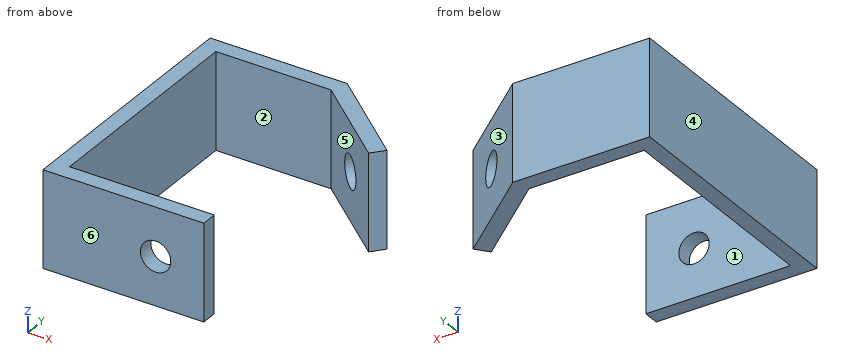
```python
from build123d import *

# Parameters (mm, degrees)
BOSS_EXTRUDE1_DEPTH = 38.1
SKETCH3_R           = 6
CUT_EXTRUDE1_DEPTH  = 23.1
SKETCH4_R           = 6.358205361
CUT_EXTRUDE2_DEPTH  = 23.1


with BuildPart() as part:
    # Sketch2 → Boss-Extrude1 (new body)
    with BuildSketch(Plane.XY):
        Polygon((0, -39.756624631), (63.51, -39.756624631), (63.51, -33.406624631), (6.35, -33.406624631), (6.35, 55.493375369), (51.808789012, 55.493375369), (84.579242619, 27.995699834), (88.66094394, 32.860082048), (54.12, 61.843375369), (0, 61.843375369), align=None)
    extrude(amount=BOSS_EXTRUDE1_DEPTH)

    # Sketch3 → Cut-Extrude1 (cut)
    with BuildSketch(Plane.XZ.offset(39.756624631)):
        with Locations(Location((44.47, 19.05, 0), (0, 0, 270))):
            Circle(SKETCH3_R)
    extrude(amount=-CUT_EXTRUDE1_DEPTH, mode=Mode.SUBTRACT)

    # Sketch4 → Cut-Extrude2 (cut)
    with BuildSketch(Plane(origin=(52.81299808, 62.940080198, 0), x_dir=(0.7660444431189768, -0.6427876096865409, 0), z_dir=(0.6427876096865408, 0.7660444431189767, 0))):
        with Locations(Location((25.986169834, -19.05, 0), (0, 0, 180))):
            Circle(SKETCH4_R)
    extrude(amount=-CUT_EXTRUDE2_DEPTH, mode=Mode.SUBTRACT)


solid = part.part
```
Check sheet for the modelled part. Datum: model origin and axes. Units: mm. Face numbers are marked on the shaded views. A direction names the side the tool comes from. Coordinates: 2 decimals unless noted, no trailing zeros. Loops run counter-clockwise (first coordinate to the right, second up) from the corner with the lowest first, then second, coordinate; pieces in that order, holes last.
1) Release check for a two-part mould opening along Y. For the marked faces 4, 5 and 6 record: released by +Y, released by -Y, zero draft, split by the parting line, or undercut.
2) Access from +Z, -Z, +X, -X, +Y, -Y to the whole of each face (thin tool, end or side, straight path). Record for the marked faces 1, 2 and 3.
3) Material ranges on probe 1 along Y at (x, z) = (51, 13.5); probe 2 along X at (y, z) = (-35, 19.05); probe 3 along Z at (x, y) = (44, -34), recorded low to high.
4) Sectioned sample at B-B (z = 21.5). Record the boundary of the cut face in (x, y) (3 decimals), and give its area (3 significant figures).
5) Sectioned sample at D-D (z = 10). Record the boundary of the cut face in (x, y).
6) Sectioned sample at C-C (y = 35.5). Record the boundary of the cut face in (x, z).
7) Gauge pin test, flat ends, axial feed: pin 1 (8 mm diameter, centred on y = 45, z = 17, fed in from +X); pin 2 (5 mm diameter, centred on y = 47.5, z = 33.5, fed in from -X); pin 3 (1.9 mm diameter, centred on y = -37.5, z = 20, fed in from +X). Record the tip position at first contact, or that the pin passes through.
8) Sectioned sample at A-A (x = 44.47). Record the boundary of the cut face in (y, z), and give its area (3 significant figures).
Check sheet entries:
1. face 4: zero draft
1. face 5: undercut
1. face 6: released by -Y
2. face 1: +Z, -Z, +X
2. face 2: +Z, -Z
2. face 3: +Z, -Z, +X, +Y
3. probe 1: y = -39.76 to -33.41, 55.49 to 61.84
3. probe 2: x = 0 to 38.47, 50.47 to 63.51
3. probe 3: z = 0 to 13.07, 25.03 to 38.1
4. outline: (0, -39.757) - (38.993, -39.757) - (38.993, -33.407) - (6.35, -33.407) - (6.35, 55.493) - (51.809, 55.493) - (64.143, 45.143) - (68.225, 50.008) - (54.12, 61.843) - (0, 61.843) - close; (49.947, -39.757) - (63.51, -39.757) - (63.51, -33.407) - (49.947, -33.407) - close; (73.132, 37.601) - (84.579, 27.996) - (88.661, 32.86) - (77.214, 42.465) - close
4. area: 1,440 mm2
5. outline: (0, -39.76) - (63.51, -39.76) - (63.51, -33.41) - (6.35, -33.41) - (6.35, 55.49) - (51.81, 55.49) - (84.58, 28) - (88.66, 32.86) - (54.12, 61.84) - (0, 61.84) - close
6. outline: (0, 0) - (6.35, 0) - (6.35, 38.1) - (0, 38.1) - close; (75.64, 0) - (85.51, 0) - (85.51, 38.1) - (75.64, 38.1) - close
7. pin 1: stops at x = 78.96
7. pin 2: stops at x = 0
7. pin 3: stops at x = 63.51
8. outline: (-39.76, 0) - (-33.41, 0) - (-33.41, 13.05) - (-39.76, 13.05) - close; (-39.76, 25.05) - (-33.41, 25.05) - (-33.41, 38.1) - (-39.76, 38.1) - close; (55.49, 0) - (61.84, 0) - (61.84, 38.1) - (55.49, 38.1) - close
8. area: 408 mm2
